```python
from build123d import *

# Parameters (mm, degrees)
CROQUIS1_R                                           = 40.5
CROQUIS1_R_2                                         = 35.5
SALIENTE_EXTRUIR1_DEPTH                              = 9
CROQUIS2_R                                           = 1.7
SALIENTE_EXTRUIR2_DEPTH                              = 2.5
REDONDEO1_R                                          = 10
CROQUIS4_R                                           = 1.7
SALIENTE_EXTRUIR3_DEPTH                              = 5
REDONDEO2_R                                          = 2
MATRIZC1_COUNT                                       = 4
REDONDEO2_OF_MATRIZC1_R                              = 2
REFRENTADO_PARA_TORNILLO_CON_CABEZA_PLAN_D           = 3.4
REFRENTADO_PARA_TORNILLO_CON_CABEZA_PLAN_CBORE_D     = 6.5
REFRENTADO_PARA_TORNILLO_CON_CABEZA_PLAN_CBORE_DEPTH = 14
CROQUIS8_R                                           = 3.25
CROQUIS8_R_2                                         = 1.7
SALIENTE_EXTRUIR4_DEPTH                              = 4
MATRIZC2_COUNT                                       = 3
MATRIZC2_ANGLE                                       = 90
SIMETR_A1_COPY_1_D                                   = 3.4
SIMETR_A1_COPY_1_CBORE_D                             = 6.5
SIMETR_A1_COPY_1_CBORE_DEPTH                         = 14
SIMETR_A1_COPY_2_D                                   = 3.4
SIMETR_A1_COPY_2_CBORE_D                             = 6.5
SIMETR_A1_COPY_2_CBORE_DEPTH                         = 14
SIMETR_A1_COPY_3_SKETCH_R                            = 3.25
SIMETR_A1_COPY_3_SKETCH_R_2                          = 1.7
SIMETR_A1_COPY_3_DEPTH                               = 4
SIMETR_A1_COPY_4_SKETCH_R                            = 3.25
SIMETR_A1_COPY_4_SKETCH_R_2                          = 1.7
SIMETR_A1_COPY_4_DEPTH                               = 4
SIMETR_A1_COPY_5_D                                   = 3.4
SIMETR_A1_COPY_5_CBORE_D                             = 6.5
SIMETR_A1_COPY_5_CBORE_DEPTH                         = 14
SIMETR_A1_COPY_6_SKETCH_R                            = 3.25
SIMETR_A1_COPY_6_SKETCH_R_2                          = 1.7
SIMETR_A1_COPY_6_DEPTH                               = 4
REDONDEO4_R                                          = 5


with BuildPart() as part:
    # Croquis1 → Saliente-Extruir1 (new, symmetric)
    with BuildSketch(Plane(origin=(0, 0, 0), x_dir=(1, 0, 0), z_dir=(0, 1, 0))):
        with Locations(Location((0, 0, 0), (0, 0, 270))):
            Circle(CROQUIS1_R)
        with Locations(Location((0, 0, 0), (0, 0, 270))):
            Circle(CROQUIS1_R_2, mode=Mode.SUBTRACT)
    extrude(amount=SALIENTE_EXTRUIR1_DEPTH, both=True)

    # Croquis2 → Saliente-Extruir2 (add, symmetric)
    with BuildSketch(Plane.XZ.offset(-9)):
        with BuildLine():
            Line((-15, 37.619808612), (-15, 57.619808612))
            Line((-15, 57.619808612), (15, 57.619808612))
            Line((15, 57.619808612), (15, 37.619808612))
            ThreePointArc((15, 37.619808612), (0, 40.5), (-15, 37.619808612))
        make_face()
        with Locations(Location((-7.5, 47.916594203, 0), (0, 0, 270))):
            Circle(CROQUIS2_R, mode=Mode.SUBTRACT)
        with Locations(Location((7.5, 47.916594203, 0), (0, 0, 90))):
            Circle(CROQUIS2_R, mode=Mode.SUBTRACT)
    extrude(amount=SALIENTE_EXTRUIR2_DEPTH, both=True)

    # Redondeo1
    redondeo1_edges = [part.edges().sort_by_distance(p)[0] for p in [
        (-15, 7.75, 37.619808612),
        (15, 7.75, 37.619808612),
        (15, 9, 57.619808612),
        (-15, 9, 57.619808612),
    ]]
    fillet(redondeo1_edges, radius=REDONDEO1_R)

    # Croquis4 → Saliente-Extruir3 (add)
    with BuildSketch(Plane(origin=(0, -6, 0), x_dir=(-1, 0, 0), z_dir=(0, -1, 0))):
        with BuildLine():
            Line((-3.75, -35.301380993), (-3.75, -28))
            Line((-3.75, -28), (3.75, -28))
            Line((3.75, -28), (3.75, -35.301380993))
            ThreePointArc((3.75, -35.301380993), (0, -35.5), (-3.75, -35.301380993))
        make_face()
        with Locations(Location((0, -31.5, 0), (0, 0, 90))):
            Circle(CROQUIS4_R, mode=Mode.SUBTRACT)
    saliente_extruir3 = extrude(amount=-SALIENTE_EXTRUIR3_DEPTH)

    # Redondeo2
    redondeo2_edges = [part.edges().sort_by_distance(p)[0] for p in [
        (-3.75, -3.5, 35.301380993),
        (3.75, -3.5, 35.301380993),
        (3.75, -3.5, 28),
        (-3.75, -3.5, 28),
    ]]
    fillet(redondeo2_edges, radius=REDONDEO2_R)

    # MatrizC1: Saliente-Extruir3 ×4 about axis
    matrizc1_axis = Axis((0, 0, 0), (0, 1, 0))
    for i in range(1, MATRIZC1_COUNT):
        add(saliente_extruir3.rotate(matrizc1_axis, i * 360 / MATRIZC1_COUNT))

    # Redondeo2 of MatrizC1
    redondeo2_of_matrizc1_edges = [part.edges().sort_by_distance(p)[0] for p in [
        (35.301380993, -3.5, 3.75),
        (35.301380993, -3.5, -3.75),
        (28, -3.5, -3.75),
        (28, -3.5, 3.75),
        (3.75, -3.5, -35.301380993),
        (-3.75, -3.5, -35.301380993),
        (-3.75, -3.5, -28),
        (3.75, -3.5, -28),
        (-35.301380993, -3.5, -3.75),
        (-35.301380993, -3.5, 3.75),
        (-28, -3.5, 3.75),
        (-28, -3.5, -3.75),
    ]]
    fillet(redondeo2_of_matrizc1_edges, radius=REDONDEO2_OF_MATRIZC1_R)

    # Refrentado para tornillo con cabeza plana de M31 (through all)
    with Locations(Plane(origin=(0, -9, 0), x_dir=(-1, 0, 0), z_dir=(0, -1, 0))):
        with Locations((0, 40.5)):
            refrentado_para_tornillo_con_cabeza_plan = CounterBoreHole(REFRENTADO_PARA_TORNILLO_CON_CABEZA_PLAN_D / 2, REFRENTADO_PARA_TORNILLO_CON_CABEZA_PLAN_CBORE_D / 2, REFRENTADO_PARA_TORNILLO_CON_CABEZA_PLAN_CBORE_DEPTH)

    # Croquis8 → Saliente-Extruir4 (add)
    with BuildSketch(Plane.XZ.offset(-5)):
        with Locations((0, -40.5)):
            Circle(CROQUIS8_R)
        with Locations(Location((0, -40.5, 0), (0, 0, 270))):
            Circle(CROQUIS8_R_2, mode=Mode.SUBTRACT)
    saliente_extruir4 = extrude(amount=-SALIENTE_EXTRUIR4_DEPTH)

    # MatrizC2: Refrentado para tornillo con cabeza plana de M31, Saliente-Extruir4 ×3 about axis
    matrizc2_axis = Axis((0, 0, 0), (0, 1, 0))
    add([refrentado_para_tornillo_con_cabeza_plan.rotate(matrizc2_axis, i * MATRIZC2_ANGLE / (MATRIZC2_COUNT - 1)) for i in range(1, MATRIZC2_COUNT)], mode=Mode.SUBTRACT)
    add([saliente_extruir4.rotate(matrizc2_axis, i * MATRIZC2_ANGLE / (MATRIZC2_COUNT - 1)) for i in range(1, MATRIZC2_COUNT)])

    # Simetría1 copy 1 (through all)
    with Locations(Plane(origin=(0, -9, 0), x_dir=(0.7071067811865467, 0, 0.7071067811865483), z_dir=(0, -1, 0))):
        with Locations((0, -40.5)):
            CounterBoreHole(SIMETR_A1_COPY_1_D / 2, SIMETR_A1_COPY_1_CBORE_D / 2, SIMETR_A1_COPY_1_CBORE_DEPTH)

    # Simetría1 copy 2 (through all)
    with Locations(Plane(origin=(0, -9, 0), x_dir=(0, 0, 1), z_dir=(0, -1, 0))):
        with Locations((0, -40.5)):
            CounterBoreHole(SIMETR_A1_COPY_2_D / 2, SIMETR_A1_COPY_2_CBORE_D / 2, SIMETR_A1_COPY_2_CBORE_DEPTH)

    # Simetría1 copy 3 sketch → Simetría1 copy 3 (add)
    with BuildSketch(Plane(origin=(0, 5, 0), x_dir=(-0.7071067811865467, 0, -0.7071067811865483), z_dir=(0, -1, 0))):
        with Locations((0, 40.5)):
            Circle(SIMETR_A1_COPY_3_SKETCH_R)
        with Locations((0, 40.5)):
            Circle(SIMETR_A1_COPY_3_SKETCH_R_2, mode=Mode.SUBTRACT)
    extrude(amount=-SIMETR_A1_COPY_3_DEPTH)

    # Simetría1 copy 4 sketch → Simetría1 copy 4 (add)
    with BuildSketch(Plane(origin=(0, 5, 0), x_dir=(0, 0, -1), z_dir=(0, -1, 0))):
        with Locations((0, 40.5)):
            Circle(SIMETR_A1_COPY_4_SKETCH_R)
        with Locations((0, 40.5)):
            Circle(SIMETR_A1_COPY_4_SKETCH_R_2, mode=Mode.SUBTRACT)
    extrude(amount=-SIMETR_A1_COPY_4_DEPTH)

    # Simetría1 copy 5 (through all)
    with Locations(Plane.XZ.offset(9)):
        with Locations((0, -40.5)):
            CounterBoreHole(SIMETR_A1_COPY_5_D / 2, SIMETR_A1_COPY_5_CBORE_D / 2, SIMETR_A1_COPY_5_CBORE_DEPTH)

    # Simetría1 copy 6 sketch → Simetría1 copy 6 (add)
    with BuildSketch(Plane(origin=(0, 5, 0), x_dir=(-1, 0, 0), z_dir=(0, -1, 0))):
        with Locations((0, 40.5)):
            Circle(SIMETR_A1_COPY_6_SKETCH_R)
        with Locations((0, 40.5)):
            Circle(SIMETR_A1_COPY_6_SKETCH_R_2, mode=Mode.SUBTRACT)
    extrude(amount=-SIMETR_A1_COPY_6_DEPTH)

    # Redondeo4
    # the kernel refuses this fillet: 5 mm, written as the material it adds along each edge
    with BuildSketch(Plane(origin=(3.247382872, 5, -40.369598765), x_dir=(-0.26298456130180026, 0, -0.9648000417272481), z_dir=(0, 1, 0)), Plane(origin=(-26.249370591, 5, -30.841863491), x_dir=(-0.8681748186382738, 0, -0.4962584853505281), z_dir=(0, 1, 0)), Plane(origin=(-40.369598765, 5, -3.247382872), x_dir=(-0.9648000417272475, 0, 0.2629845613018025), z_dir=(0, 1, 0)), Plane(origin=(30.841863491, 5, -26.249370591), x_dir=(0.49625848535052886, 0, -0.8681748186382734), z_dir=(0, 1, 0)), Plane(origin=(40.369598765, 5, 3.247382872), x_dir=(0.9648000417272491, 0, -0.2629845613017969), z_dir=(0, 1, 0))) as redondeo4_piece_1:
        with BuildLine():
            CenterArc((3.467064855, -4.767356337), REDONDEO4_R, 107.546751442, 48.438780652)
            ThreePointArc((-1.100148756, -2.732519778), (-0.525223225, -1.376265293), (0, 0))
            ThreePointArc((0, 0), (0.979822677, -0.151218381), (1.959645353, 0))
        make_face()
    extrude(amount=4)
    with BuildSketch(Plane(origin=(-3.247382872, 5, -40.369598765), x_dir=(-0.9932049358227855, 0, 0.11637850083781144), z_dir=(0, 1, 0)), Plane(origin=(-30.841863491, 5, -26.249370591), x_dir=(-0.6200099181014976, 0, 0.7845939723549846), z_dir=(0, 1, 0)), Plane(origin=(26.249370591, 5, -30.841863491), x_dir=(-0.784593972354982, 0, -0.6200099181015007), z_dir=(0, 1, 0)), Plane(origin=(40.369598765, 5, -3.247382872), x_dir=(-0.1163785008378116, 0, -0.9932049358227855), z_dir=(0, 1, 0))) as redondeo4_piece_2:
        with BuildLine():
            CenterArc((3.127505063, -4.99669263), REDONDEO4_R, 92.084097226, 48.438780652)
            ThreePointArc((-0.731887458, -1.817842308), (-0.22566775, -0.965398127), (0, 0))
            ThreePointArc((0, 0), (1.472836687, -0.026789699), (2.945673373, 0))
        make_face()
    extrude(amount=4)
    with BuildSketch(Plane(origin=(-40.369598765, 5, 3.247382872), x_dir=(-0.9648000417272488, 0, -0.262984561301798), z_dir=(0, 1, 0))) as redondeo4_piece_3:
        with BuildLine():
            CenterArc((3.467064855, 4.767356337), REDONDEO4_R, 204.014467906, 48.438780652)
            ThreePointArc((-1.100148756, 2.732519778), (-0.525223225, 1.376265293), (0, 0))
            ThreePointArc((0, 0), (0.979822677, 0.151218381), (1.959645353, 0))
        make_face()
    extrude(amount=4)


solid = part.part
```
Can you work these out from the model? Positions are in its coordinate system, mm. A direction names the side the tool comes from. Coordinates: 2 decimals unless noted, no trailing zeros. Loops run counter-clockwise (first coordinate to the right, second up) from the corner with the lowest first, then second, coordinate; pieces in that order, holes last. Notation, with made-up numbers: (71, 87.25) -> (103, 87.25) arc R30 cw to (103, 118.25) -> close; hole circle Ø2 at (-4, -37.75). An arc over 180 degrees is marked (long way). Put each result on its own line as item: value. Start each with the question number.
Q1. I want a section at A-A (x = 0). Count the separate pieces of the cut face and the enclosed holes in it, plus the area to 3 significant figures.
Q2. I want a section at D-D (z = -14.5). Write out the boundary of the cut face in (x, y), plus the area to 3 significant figures.
Q3. I want a section at B-B (z = 22.5). Write out the boundary of the cut face in (x, y), plus the area to 3 significant figures.
Q4. If I drill on line 1 (Z direction, x = -31.5, y = -3.4), over which ranges is the centre line in solid material (lowest first)? Write a range as [from, to].
Q5. I want a section at C-C (x = 18.5). Write out the boundary of the cut face in (y, z), plus the area to 3 significant figures.
Q6. Thinking about a two-plate mould opening in Z: for faces 1 (the face through (0, 6.5, 47)), 2 (the face through (-15.3, 0.1, -37.5)), 3 (the face through (34.55, -3.46, 4.48)), 4 (the face through (-40.758, 6.972, 4.238)), which applies, pulls with the +Z half, pulls with the -Z half, needs draft (parallel to the pull), parting line crosses it, or undercut?
Q7. For faces 5 (the face through (-37.25, -2.1, -0.07)), 6 (the face through (-12.15, 9.04, 54.61)), 7 (the face through (37.5, 0.1, -15.3)), 8 (the face through (34.55, -3.46, -4.48)), 9 (the face through (0, 9, 57.62)), which set-ups out of +Z, -Z, +X, -X, +Y, -Y let a thin tool reach every point of the face, with its end or its side?
Q8. I'm going to push flat-ended pins straight in: P1, Ø11, axis at x = -0.5, z = 49.5, coming from the -Y side; P2, Ø10, axis at x = 17.5, z = -31.5, coming from the +Y side; P3, Ø4, axis at x = 2.5, z = 33, coming from the +Y side; P4, Ø2, axis at x = 7.5, z = 47.92, coming from the -Y side. Where does each tip first touch, or does it pass through?
Taken from the geometry:
1. separate pieces: 5
1. enclosed holes: 0
1. area: 260 mm2
2. outline: (-37.82, -9) -> (-32.4, -9) -> (-32.4, 9) -> (-37.82, 9) -> close; (32.4, -9) -> (37.82, -9) -> (37.82, 9) -> (32.4, 9) -> close
2. area: 195 mm2
3. outline: (-33.67, -9) -> (-27.46, -9) -> (-27.46, 9) -> (-33.67, 9) -> close; (27.46, -9) -> (33.67, -9) -> (33.67, 9) -> (27.46, 9) -> close
3. area: 224 mm2
4. line 1: z = [-25.46, -16.37], [-3.75, -1.7], [1.7, 3.75], [16.37, 25.46]
5. outline: (-9, -36.03) -> (9, -36.03) -> (9, -30.3) -> (-9, -30.3) -> close; (-9, 30.3) -> (9, 30.3) -> (9, 36.28) -> (6.5, 36.28) -> (6.5, 36.03) -> (-9, 36.03) -> close
5. area: 207 mm2
6. face 1: needs draft
6. face 2: pulls with the -Z half
6. face 3: undercut
6. face 4: pulls with the +Z half
7. face 5: -X, -Y
7. face 6: +Z, -X, +Y, -Y
7. face 7: -Z, +X, -Y
7. face 8: +Y, -Y
7. face 9: +Z, +X, -X, +Y, -Y
8. P1: stops at y = 6.5
8. P2: stops at y = 9
8. P3: stops at y = -1
8. P4: passes through
